from build123d import *

# Parameters (mm, degrees)
SKETCH_1_R               = 55
EXTRUDE_1_DEPTH          = 62
EXTRUDE_2_DEPTH          = 35
SKETCH_3_R               = 37
CUT_EXTRUDE_1_DEPTH      = 63
CUT_EXTRUDE_1_DEPTH_BACK = 63
SKETCH_4_R               = 45
CUT_EXTRUDE_2_DEPTH      = 30
CUT_EXTRUDE_3_REACH      = 161
SKETCH_6_R               = 19.352
CHAMFER_2_SIZE           = 1.648
SKETCH_9_R               = 2.4455
CUT_EXTRUDE_5_DEPTH      = 18
CHAMFER_3_SIZE           = 0.5545


with BuildPart() as part:
    # Эскиз1 → Бобышка-Вытянуть1 (new body, symmetric)
    with BuildSketch(Plane.XY):
        Circle(SKETCH_1_R)
    extrude(amount=EXTRUDE_1_DEPTH, both=True)

    # Эскиз2 → Бобышка-Вытянуть2 (add, symmetric)
    with BuildSketch(Plane.XY):
        Polygon((-104, 0), (-104, 35), (-10.947280704, 53.899508766), (-10.947280704, 0), align=None)
    extrude_2 = extrude(amount=EXTRUDE_2_DEPTH, both=True)

    # Зеркальное отражение1: Бобышка-Вытянуть2 across plane
    add(extrude_2.mirror(Plane(origin=(-104, 0, 35), x_dir=(0, 0, 1), z_dir=(0, 1, 0))))

    # Эскиз3 → Вырез-Вытянуть1 (cut, two sides)
    with BuildSketch(Plane.XY) as cut_extrude_1_sk:
        Circle(SKETCH_3_R)
    extrude(amount=CUT_EXTRUDE_1_DEPTH, mode=Mode.SUBTRACT)
    extrude(cut_extrude_1_sk.sketch, amount=-CUT_EXTRUDE_1_DEPTH_BACK, mode=Mode.SUBTRACT)

    # Эскиз4 → Вырез-Вытянуть2 (cut)
    with BuildSketch(Plane.XY.offset(62)):
        Circle(SKETCH_4_R)
    cut_extrude_2 = extrude(amount=-CUT_EXTRUDE_2_DEPTH, mode=Mode.SUBTRACT)

    # Зеркальное отражение2: Вырез-Вытянуть2 across plane
    add(cut_extrude_2.mirror(Plane.XY), mode=Mode.SUBTRACT)

    # Эскиз6 → Вырез-Вытянуть3 (cut, up to next)
    with BuildSketch(Plane.ZY.offset(104), mode=Mode.PRIVATE) as cut_extrude_3_sk1:
        Circle(SKETCH_6_R)
    cut_extrude_3_tool1 = extrude(cut_extrude_3_sk1.sketch, amount=-CUT_EXTRUDE_3_REACH, mode=Mode.PRIVATE) & part.part
    add(cut_extrude_3_tool1.solids().sort_by_distance((-104, 0, 0))[0], mode=Mode.SUBTRACT)

    # Фаска2
    chamfer_2_edges = [part.edges().sort_by_distance(p)[0] for p in [
        (-104, 0, -19.352),
    ]]
    chamfer(chamfer_2_edges, length=CHAMFER_2_SIZE)

    # Эскиз9 → Вырез-Вытянуть5 (cut)
    with BuildSketch(Plane(origin=(0, 0, -62), x_dir=(-1, 0, 0), z_dir=(0, 0, -1))):
        with Locations((45, 0)):
            Circle(SKETCH_9_R)
    cut_extrude_5 = extrude(amount=-CUT_EXTRUDE_5_DEPTH, mode=Mode.SUBTRACT)

    # Зеркальное отражение3: Вырез-Вытянуть5 across plane
    add(cut_extrude_5.mirror(Plane.XY), mode=Mode.SUBTRACT)

    # Фаска3
    chamfer_3_edges = [part.edges().sort_by_distance(p)[0] for p in [
        (-47.4455, 0, -62),
        (-47.4455, 0, 62),
    ]]
    chamfer(chamfer_3_edges, length=CHAMFER_3_SIZE)


solid = part.part
Input: part model. Units: mm. Frame: model coordinates. A direction names the side the tool comes from. Round coordinates to 2 decimals unless told otherwise and drop trailing zeros. Order: outer loops, then holes, each group sorted by start corner. A loop starts at its lowest first (then second) coordinate and runs counter-clockwise, first axis right, second up.
1. Material intervals for line 1 (X direction, y = 0, z = -42); line 2 (Z direction, x = -96, y = -0.5); line 3 (Y direction, x = 0, z = -12.5), sorted ascending.
The answers:
line 1: x = -55 to -45, 45 to 55
line 2: z = -35 to -19.35, 19.35 to 35
line 3: y = -55 to -37, 37 to 55
2. Cut plane D-D, the plane y = 32. Output: boundary loops of the cut face in (x, z).
The answers:
outline: (-104, -35) - (-44.73, -35) - (-44.73, -62) - (-31.64, -62) - (-31.64, -32) - (-18.57, -32) - (-18.57, 32) - (-31.64, 32) - (-31.64, 62) - (-44.73, 62) - (-44.73, 35) - (-104, 35) - close; (18.57, -32) - (31.64, -32) - (31.64, -62) - (44.73, -62) - (44.73, 62) - (31.64, 62) - (31.64, 32) - (18.57, 32) - close
3. Cut plane A-A, the plane y = 0. State how many separate pieces and enclosed holes the cut face has, then the cut area to 3 significant figures.
The answers:
separate pieces: 3
enclosed holes: 0
area: 4,250 mm2
4. Pin query (flat end, axial travel): P1, Ø12, axis at y = -37, z = 25, coming from the +X side; P2, Ø2, axis at x = -6.5, z = 29.5, coming from the -Y side; P3, Ø3, axis at y = 3, z = -7.5, coming from the -X side. Return the tip coordinate at first contact, or that it passes through.
The answers:
P1: stops at x = 45.43
P2: stops at y = -54.72
P3: stops at x = 36.73
5. Cut plane B-B, the plane x = 0. Output: boundary loops of the cut face in (y, z), then the cut area to 3 significant figures.
The answers:
outline: (-55, -62) - (-45, -62) - (-45, -32) - (-37, -32) - (-37, 32) - (-45, 32) - (-45, 62) - (-55, 62) - close; (37, -32) - (45, -32) - (45, -62) - (55, -62) - (55, 62) - (45, 62) - (45, 32) - (37, 32) - close
area: 3,500 mm2
6. Set-up query: faces 4 (the face through (-67.44, 0.851, -19.333)), 5 (the face through (-104, -15, 16)), 6 (the face through (34.18, -14.17, 0.45)), 7 (the face through (-10, -36, 32)), 8 (the face through (-47.445, -0.055, -52.845)). Return all of +Z, -Z, +X, -X, +Y, -Y with unobstructed straight access to the full face (end or side cutting, diameter ignored); none if empty.
The answers:
face 4: -X
face 5: +Z, -Z, -X, +Y, -Y
face 6: +Z, -Z
face 7: +Z
face 8: -Z
7. Mould query, pull axis Y, two halves, no side actions, for faces 1 (the face through (52.46, 16.52, 0.87)), 2 (the face through (-4, 45, -62)), 3 (the face through (41.569, -17.235, 47.21)). Classes: released by +Y, released by -Y, zero draft, split by the parting line, or undercut.
The answers:
face 1: split by the parting line
face 2: zero draft
face 3: undercut
8. Cut plane C-C, the plane z = 0. Output: boundary loops of the cut face in (x, y), then the cut area to 3 significant figures.
The answers:
outline: (-104, -35) - (-10.95, -53.9) arc R55 ccw (long way) to (-10.95, 53.9) - (-104, 35) - (-104, 21) - (-102.35, 19.35) - (-31.54, 19.35) arc R37 cw (long way) to (-31.54, -19.35) - (-102.35, -19.35) - (-104, -21) - close
area: 7,260 mm2
